Verification items for the finished model (mm, model axes). Face numbers are marked on the shaded views. A direction names the side the tool comes from. Round coordinates to 2 decimals unless told otherwise and drop trailing zeros. Loops run counter-clockwise (first coordinate to the right, second up) from the corner with the lowest first, then second, coordinate; pieces in that order, holes last. Notation, with made-up numbers: (-3, -11) -> (9, -11) arc R31 ccw to (9, 20) -> close; hole circle Ø5 at (43, 87.25). An arc over 180 degrees is marked (long way). Write item = value, one per line.
```python
from build123d import *

# Parameters (mm, degrees)
PLATE_DEPTH  = 1
PILLAR_START = -7
PILLAR_DEPTH = 7
CUT_DEPTH    = 12.862454801607791
HOLESKE_R    = 0.4249999999999999
HOLE_DEPTH   = 11.491832758845009
FILLET_2_R   = 0.5


with BuildPart() as part:
    # PlateSke → Plate (new body)
    with BuildSketch(Plane.XY):
        with BuildLine():
            Line((-4.829949748426477, -0.8255818721816728), (-0.8500000000000022, 1.472243186433545))
            ThreePointArc((-0.8500000000000022, 1.472243186433545), (1e-16, 1.7000000000000004), (0.8500000000000022, 1.472243186433545))
            Line((0.8500000000000022, 1.472243186433545), (4.829949748426477, -0.8255818721816728))
            ThreePointArc((4.829949748426477, -0.8255818721816728), (3e-16, -4.899999999999999), (-4.829949748426477, -0.8255818721816728))
        make_face()
        Polygon((1.0392304845413274, 0), (0.5196152422706616, 0.9000000000000019), (-0.5196152422706678, 0.8999999999999982), (-1.0392304845413274, -7.26e-15), (-0.5196152422706553, -0.9000000000000056), (0.5196152422706742, -0.8999999999999948), align=None, mode=Mode.SUBTRACT)
    extrude(amount=PLATE_DEPTH)

    # PillarSke → Pillar (add)
    with BuildSketch(Plane.XY.offset(1).offset(PILLAR_START)):
        with BuildLine():
            Line((-6.641372894228101, -1.87140751302655), (-4.829949748426477, -0.8255818721816716))
            ThreePointArc((-4.829949748426477, -0.8255818721816716), (-1.88e-15, -4.899999999999999), (4.829949748426477, -0.8255818721816728))
            Line((4.829949748426477, -0.8255818721816728), (6.641372894228101, -1.8714075130265588))
            ThreePointArc((6.641372894228101, -1.8714075130265588), (-4.17e-15, -6.8999999999999995), (-6.641372894228101, -1.87140751302655))
        make_face()
    extrude(amount=PILLAR_DEPTH)

    # CutSke → Cut (cut, through all)
    with BuildSketch(Plane.XY.offset(1)):
        with BuildLine():
            Line((-1.3444863728671024, -1.7000000000000057), (1.3444863728670877, -1.700000000000006))
            Line((1.3444863728670877, -1.700000000000006), (5.53527589923164, -4.119553461163642))
            ThreePointArc((5.53527589923164, -4.119553461163642), (-2.64e-15, -6.899999999999998), (-5.5352758992316415, -4.119553461163638))
            Line((-5.5352758992316415, -4.119553461163638), (-1.3444863728671024, -1.7000000000000057))
        make_face()
    extrude(amount=-CUT_DEPTH, mode=Mode.SUBTRACT)

    # HoleSke → Hole (cut, through all)
    with BuildSketch(Plane(origin=(0, 0, -6), x_dir=(-1, 0, 0), z_dir=(0, 0, -1))):
        with Locations((-5.317327275986198, -2.5381645669665653)):
            Circle(HOLESKE_R)
        with Locations(Location((5.317327275986198, -2.5381645669665653, 0), (0, 0, 180))):
            Circle(HOLESKE_R)
    extrude(amount=-HOLE_DEPTH, mode=Mode.SUBTRACT)

    # Fillet 2
    fillet_2_edges = [part.edges().sort_by_distance(p)[0] for p in [
        (-4.829949748426477, -0.8255818721816717, -3),
        (6.641372894228101, -1.8714075130265588, -2.5),
        (-6.641372894228101, -1.8714075130265502, -2.5),
        (4.829949748426477, -0.8255818721816734, -3),
        (-1.3444863728671024, -1.7000000000000057, 0.5),
        (-5.535275899231642, -4.119553461163638, -2.5),
        (1.3444863728670877, -1.700000000000006, 0.5),
        (-3.7865857210858582, -3.1099467160819145, -3),
        (3.7865857210858542, -3.1099467160819194, -3),
        (5.535275899231641, -4.119553461163642, -2.5),
    ]]
    fillet(fillet_2_edges, radius=FILLET_2_R)


solid = part.part
```
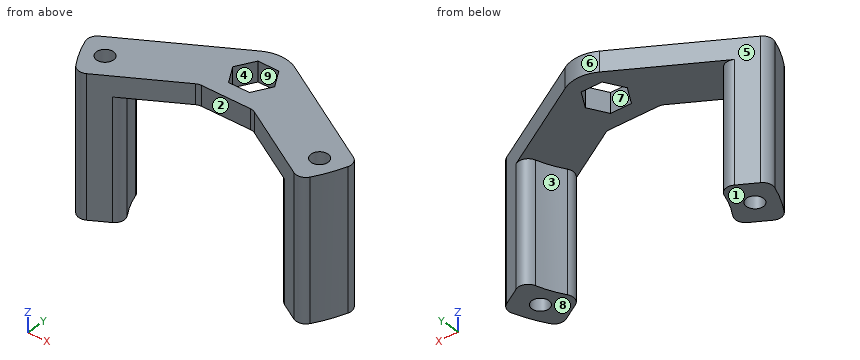
(1) Set-up check for the marked faces 1, 2, 3, 4 and 5: record each of +Z, -Z, +X, -X, +Y, -Y from which the full face is reachable in a straight line by a thin tool's end or side.
Filled sheet:
face_1 = -Z, +X, -X, +Y, -Y
face_2 = +Z, -Z, -Y
face_3 = -Z, +Y
face_4 = +Z, -Z
face_5 = +Z, -Z, -X, +Y
(2) Go/stop test with flat-tipped pins: pin 1 Ø0.5 at (x, z) = (0, 0.5) entering from -Y; pin 2 Ø1.5 at (x, z) = (-4.5, -1) entering from -Y; pin 3 Ø2 at (x, z) = (0, -2) entering from +Y; pin 4 Ø4 at (x, z) = (2.5, -3) entering from +Y. Record where each tip stops, or that it passes through.
Filled sheet:
pin_1 = -1.7
pin_2 = -3.94
pin_3 = through
pin_4 = -1.94
(3) Sectioned sample at B-B, the plane x = -0.25. Record the cut outline in (y, z), and give its area (3 significant figures).
Filled sheet:
outline = (-1.7, 0) -> (-0.9, 0) -> (-0.9, 1) -> (-1.7, 1) -> close; (0.9, 0) -> (1.68, 0) -> (1.68, 1) -> (0.9, 1) -> close
area = 1.58 mm2
(4) Material ranges on probe 1 along X at (y, z) = (-2.4, 0.75); probe 2 along Z at (x, y) = (2.75, -0.4); probe 3 along X at (y, z) = (-2.9, -4.75), recorded low to high. Write a range as from..to.
Filled sheet:
probe_1 = -6.47..-5.72, -4.92..-2.56, 2.56..4.92, 5.72..6.47
probe_2 = 0..1
probe_3 = -6.26..-5.54, -5.09..-4.02, 4.02..5.09, 5.54..6.26
(5) Draft check along X on the marked faces 6, 7, 8 and 9. Enter one of: released by +X, released by -X, zero draft, split by the parting line, or undercut.
Filled sheet:
face_6 = split by the parting line
face_7 = undercut
face_8 = zero draft
face_9 = undercut
(6) Sectioned sample at C-C, the plane y = 0.4. Record the cut outline in (x, z).
Filled sheet:
outline = (-2.71, 0) -> (-0.81, 0) -> (-0.81, 1) -> (-2.71, 1) -> close; (0.81, 0) -> (2.71, 0) -> (2.71, 1) -> (0.81, 1) -> close
(7) Sectioned sample at D-D, the plane y = -1.3. Record the cut outline in (x, z).
Filled sheet:
outline = (-5.65, -6) -> (-4.75, -6) -> (-4.75, 0) -> (4.75, 0) -> (4.75, -6) -> (5.65, -6) -> (5.65, 1) -> (-5.65, 1) -> close
(8) Sectioned sample at A-A, the plane z = -0.75. Record the cut outline in (x, y) (3 decimals).
Filled sheet:
outline = (-6.516, -2.268) arc R6.9 ccw to (-5.807, -3.726) arc R0.5 ccw to (-5.136, -3.889) -> (-4.269, -3.389) arc R0.5 ccw to (-4.101, -2.682) arc R4.9 cw to (-4.682, -1.446) arc R0.5 ccw to (-5.41, -1.16) -> (-6.294, -1.671) arc R0.5 ccw to start; (4.101, -2.682) arc R0.5 ccw to (4.269, -3.389) -> (5.136, -3.889) arc R0.5 ccw to (5.807, -3.726) arc R6.9 ccw to (6.516, -2.268) arc R0.5 ccw to (6.294, -1.671) -> (5.41, -1.16) arc R0.5 ccw to (4.682, -1.446) arc R4.9 cw to start; hole circle Ø0.85 at (-5.317, -2.538); hole circle Ø0.85 at (5.317, -2.538)
